```python
from build123d import *

# Parameters (mm, degrees)
F0_W      = 834.7400754492
F0_H      = 50.8
F1_DEPTH  = 3.048
F3_W      = 57.9247
F3_H      = 5.08
F3_W_2    = 115.8494
F3_H_2    = 3.1496
F4_DEPTH  = 3.048
F6_DEPTH  = 3.048
F7_DEPTH  = 3.049
F9_W      = 6.096
F9_H      = 6.096
F9_R      = 2.8702
F9_R_2    = 4.953
F9_R_3    = 7.9375
F10_DEPTH = 3.049
F11_DEPTH = 25.4
F12_W     = 38.1
F12_H     = 5.08
F12_H_2   = 3.1496
F13_DEPTH = 3.048


# Not quite as in the source:
# - a feature names something its author has since deleted; it is built from what else it names


with BuildPart() as f1:
    # F0 (on Front) → F1 (new body)
    with BuildSketch(Plane.XZ):
        with Locations((417.3700377246, 25.4)):
            Rectangle(F0_W, F0_H)
    extrude(amount=F1_DEPTH)

    # F3 (on face) → F4 (join)
    with BuildSketch(Plane.XZ.offset(3.048)):
        with Locations((28.96235, 53.34)):
            Rectangle(F3_W, F3_H)
        with Locations((139.1233459082, 53.34)):
            Rectangle(F3_W_2, F3_H)
        with Locations((278.2466918164, 53.34)):
            Rectangle(F3_W_2, F3_H)
        with Locations((417.3700377246, 53.34)):
            Rectangle(F3_W_2, F3_H)
        with Locations((556.4933836328, 53.34)):
            Rectangle(F3_W_2, F3_H)
        with Locations((695.616729541, 53.34)):
            Rectangle(F3_W_2, F3_H)
        with Locations((805.7777254492, 53.34)):
            Rectangle(F3_W, F3_H)
        with Locations((28.96235, -1.5748)):
            Rectangle(F3_W, F3_H_2)
        with Locations((139.1233459082, -1.5748)):
            Rectangle(F3_W_2, F3_H_2)
        with Locations((278.2466918164, -1.5748)):
            Rectangle(F3_W_2, F3_H_2)
        with Locations((417.3700377246, -1.5748)):
            Rectangle(F3_W_2, F3_H_2)
        with Locations((556.4933836328, -1.5748)):
            Rectangle(F3_W_2, F3_H_2)
        with Locations((695.616729541, -1.5748)):
            Rectangle(F3_W_2, F3_H_2)
        with Locations((805.7777254492, -1.5748)):
            Rectangle(F3_W, F3_H_2)
    extrude(amount=-F4_DEPTH)

    # F5 (on face) → F6 (join)
    with BuildSketch(Plane.XZ.offset(3.048)):
        Polygon((-6.35, 6.35), (0, 6.35), (0, 44.45), (-6.35, 44.45), (-9.525, 47.625), (-9.525, 3.175), align=None)
    extrude(amount=-F6_DEPTH)

    # F5 (on face) → F7 (cut, through all)
    with BuildSketch(Plane.XZ.offset(3.048)):
        Polygon((828.3900754492, 7.3152), (834.7400754492, 7.3152), (834.7400754492, 45.4152), (828.3900754492, 45.4152), (825.2150754492, 48.5902), (825.2150754492, 4.1402), align=None)
    extrude(amount=-F7_DEPTH, mode=Mode.SUBTRACT)

    # F9 (on face) → F10 (cut, through all)
    with BuildSketch(Plane.XZ.offset(3.048)):
        with Locations((256.3264918164, 15.621)):
            Rectangle(F9_W, F9_H)
        with Locations((278.2466918164, 15.621)):
            Rectangle(F9_W, F9_H)
        with Locations((300.1668918164, 15.621)):
            Rectangle(F9_W, F9_H)
        with Locations((235.7016918164, 15.621)):
            Circle(F9_R)
        with Locations((323.9666918164, 15.621)):
            Circle(F9_R_2)
        with Locations((278.2466918164, 34.671)):
            Circle(F9_R_3)
    extrude(amount=-F10_DEPTH, mode=Mode.SUBTRACT)

    # F8 (on face) → F11 (cut)
    with BuildSketch(Plane.XZ.offset(3.048)):
        Polygon((411.0200377246, 6.35), (417.3700377246, 6.35), (417.3700377246, 44.45), (411.0200377246, 44.45), (407.8450377246, 47.625), (407.8450377246, 3.175), align=None)
    extrude(amount=-F11_DEPTH, mode=Mode.SUBTRACT)

    # F12 (on face) → F13 (cut, through all)
    with BuildSketch(Plane.XZ.offset(3.048)):
        with Locations((139.1233459082, 53.34)):
            Rectangle(F12_W, F12_H)
        with Locations((278.2466918164, 53.34)):
            Rectangle(F12_W, F12_H)
        with Locations((417.3700377246, 53.34)):
            Rectangle(F12_W, F12_H)
        with Locations((556.4933836328, 53.34)):
            Rectangle(F12_W, F12_H)
        with Locations((695.616729541, 53.34)):
            Rectangle(F12_W, F12_H)
        with Locations((834.7400754492, 53.34)):
            Rectangle(F12_W, F12_H)
        with Locations((0, 53.34)):
            Rectangle(F12_W, F12_H)
        with Locations((0, -1.5748)):
            Rectangle(F12_W, F12_H_2)
        with Locations((139.1233459082, -1.5748)):
            Rectangle(F12_W, F12_H_2)
        with Locations((278.2466918164, -1.5748)):
            Rectangle(F12_W, F12_H_2)
        with Locations((417.3700377246, -1.5748)):
            Rectangle(F12_W, F12_H_2)
        with Locations((556.4933836328, -1.5748)):
            Rectangle(F12_W, F12_H_2)
        with Locations((695.616729541, -1.5748)):
            Rectangle(F12_W, F12_H_2)
        with Locations((834.7400754492, -1.5748)):
            Rectangle(F12_W, F12_H_2)
    extrude(amount=-F13_DEPTH, mode=Mode.SUBTRACT)


solid = f1.part
```
The listing builds one solid part. Answer for the finished solid, in the listing's coordinates (mm). Round coordinates to 2 decimals unless told otherwise and drop trailing zeros. Order: outer loops, then holes, each group sorted by start corner. A loop starts at its lowest first (then second) coordinate and runs counter-clockwise, first axis right, second up. Notation, with made-up numbers: (-25.75, 57) -> (28.25, 57) arc R16 cw to (28.25, 83) -> close; hole circle Ø8 at (61.5, -26). An arc over 180 degrees is marked (long way). Answer as CSV lines item,"result". Start each with the question number.
(1) Find the intervals of material crossed by probe 1 along X at (y, z) = (-2.3, 44.5) (3 decimals); probe 2 along X at (y, z) = (-2.9, 40.5) (3 decimals); probe 3 along Z at (x, y) = (552, -0.85), in increasing order. Write a range as from..to.
(2) The part is cut by section A-A (x = 770). Determine the outline of the cut face in (y, z), then the cut area to 3 significant figures.
(3) Flat-ended cylindrical pins translate along their axes: pin 1 Ø1.5 at (y, z) = (-1, -1.5) entering from -X; pin 2 Ø0.9 at (x, y) = (829.5, -2) entering from -Z; pin 3 Ø4 at (x, z) = (260, 3) entering from +Y; pin 4 Ø1.5 at (y, z) = (-1, -1) entering from +X. Find the tip coordinate at first contact, or state that the pin passes through.
(4) For a pull along Z with two mould halves and no side action, classify faces 1 (the face through (407, 0, 27)), 2 (the face through (270.317, -1.545, 35.02)) as +Z half, -Z half, draft (parallel to the pull), parting line (faces both ways), or undercut.
(5) The part is cut by section B-B (y = -1.1). Count the separate pieces of the cut face and the enclosed holes in it, then the cut area to 3 significant figures.
Evaluation:
1,probe 1,"-9.525..-6.4, 0..407.845, 410.97..825.215"
1,probe 2,"-9.525..272.859, 283.634..407.845, 417.37..825.215"
1,probe 3,"0..50.8"
2,outline,"(-3.05, 0) -> (0, 0) -> (0, 50.8) -> (-3.05, 50.8) -> close"
2,area,"155 mm²"
3,pin 1,"x = 19.05"
3,pin 2,"z = 0"
3,pin 3,"y = 0"
3,pin 4,"x = 815.69"
4,face 1,"draft"
4,face 2,"undercut"
5,separate pieces,"1"
5,enclosed holes,"7"
5,area,"45,500 mm²"
